from build123d import *

# Parameters (mm, degrees)
SKETCH_1_R          = 39
EXTRUDE_1_DEPTH     = 53.8
SKETCH_2_R          = 2
CUT_EXTRUDE_1_DEPTH = 3
SKETCH_3_R          = 5.25
EXTRUDE_2_DEPTH     = 20
CUT_EXTRUDE_START   = -10
SKETCH_4_R          = 5.5
SKETCH_4_R_2        = 5.25
CUT_EXTRUDE_2_DEPTH = 10
CHAMFER_1_SIZE      = 0.5
CUT_EXTRUDE_3_DEPTH = 10
CHAMFER_2_SIZE      = 1.5
SKETCH_7_W          = 5
SKETCH_7_H          = 9
CUT_EXTRUDE_4_DEPTH = 10
SKETCH_8_W          = 0.130242645
SKETCH_8_H          = 3.5
SKETCH_9_R          = 1.5
CUT_EXTRUDE_5_DEPTH = 10


with BuildPart() as part:
    # 草图1 → 凸台-拉伸1 (new body)
    with BuildSketch(Plane.XY):
        with Locations(Location((0, 0, 0), (0, 0, 180))):
            Circle(SKETCH_1_R)
    extrude(amount=EXTRUDE_1_DEPTH)

    # 草图2 → 切除-拉伸1 (cut)
    with BuildSketch(Plane.XY.offset(53.8)):
        with Locations((0, 20)):
            Circle(SKETCH_2_R)
        with Locations((17.320508076, -10)):
            Circle(SKETCH_2_R)
        with Locations((-17.320508076, -10)):
            Circle(SKETCH_2_R)
    extrude(amount=-CUT_EXTRUDE_1_DEPTH, mode=Mode.SUBTRACT)

    # 草图3 → 凸台-拉伸2 (add)
    with BuildSketch(Plane.XY.offset(53.8)):
        Circle(SKETCH_3_R)
    extrude(amount=EXTRUDE_2_DEPTH)

    # 草图4 → 切除-拉伸2 (cut)
    with BuildSketch(Plane.XY.offset(53.8).offset(CUT_EXTRUDE_START)):
        Circle(SKETCH_4_R)
        Circle(SKETCH_4_R_2, mode=Mode.SUBTRACT)
    extrude(amount=CUT_EXTRUDE_2_DEPTH, mode=Mode.SUBTRACT)

    # 倒角1
    chamfer_1_edges = [part.edges().sort_by_distance(p)[0] for p in [
        (-5.25, 0, 73.8),
    ]]
    chamfer(chamfer_1_edges, length=CHAMFER_1_SIZE)

    # 草图5 → 切除-拉伸3 (cut)
    with BuildSketch(Plane.XY.offset(73.8)):
        Polygon((4.75, 0), (4.75, 11.306536843), (10.594936623, 11.306536843), (10.594936623, -9.408936254), (4.75, -9.408936254), align=None)
    extrude(amount=-CUT_EXTRUDE_3_DEPTH, mode=Mode.SUBTRACT)

    # 倒角2
    chamfer_2_edges = [part.edges().sort_by_distance(p)[0] for p in [
        (39, 0, 53.8),
    ]]
    chamfer(chamfer_2_edges, length=CHAMFER_2_SIZE)

    # 草图6 → 切除-旋转1 (revolve, cut)
    with BuildSketch(Plane(origin=(0, 0, 0), x_dir=(1, 0, 0), z_dir=(0, 1, 0)), mode=Mode.PRIVATE) as cut_revolve_1_sk:
        Polygon((-39, 0), (-39, -1.5), (-33.508685112, 0), align=None)
    revolve(cut_revolve_1_sk.sketch.rotate(Axis((0, 0, 0), (0, 0, -1)), 154.791234703), axis=Axis((0, 0, 0), (0, 0, -1)), mode=Mode.SUBTRACT)

    # 草图7 → 切除-拉伸4 (cut)
    with BuildSketch(Plane(origin=(40, 0, 0), x_dir=(0, 0, -1), z_dir=(1, 0, 0))):
        with Locations((-7, 0)):
            Rectangle(SKETCH_7_W, SKETCH_7_H)
    extrude(amount=-CUT_EXTRUDE_4_DEPTH, mode=Mode.SUBTRACT)

    # 草图8 → 切除-旋转2 (revolve, cut)
    with BuildSketch(Plane(origin=(0, 0, 0), x_dir=(1, 0, 0), z_dir=(0, 1, 0)), mode=Mode.PRIVATE) as cut_revolve_2_sk:
        with Locations((38.934878678, -11.25)):
            Rectangle(SKETCH_8_W, SKETCH_8_H)
    revolve(cut_revolve_2_sk.sketch.rotate(Axis((0, 0, 0), (0, 0, 1)), 25.208765297), axis=Axis((0, 0, 0), (0, 0, 1)), mode=Mode.SUBTRACT)

    # 草图9 → 切除-拉伸5 (cut)
    with BuildSketch(Plane(origin=(4.75, 0, 0), x_dir=(0, 0, -1), z_dir=(1, 0, 0))):
        with Locations((-70.8, 0)):
            Circle(SKETCH_9_R)
    extrude(amount=-CUT_EXTRUDE_5_DEPTH, mode=Mode.SUBTRACT)


solid = part.part
Here's how the part is built. I have some questions about the finished solid (model axes, mm). A direction names the side the tool comes from. Round coordinates to 2 decimals unless told otherwise and drop trailing zeros. Order: outer loops, then holes, each group sorted by start corner. A loop starts at its lowest first (then second) coordinate and runs counter-clockwise, first axis right, second up. Notation, with made-up numbers: (-23, 44) -> (-10, 44) arc R22 ccw to (-10, 59) -> close; hole circle Ø11 at (37.5, 45.25). An arc over 180 degrees is marked (long way). Return JSON: item names as keys, results as strings.
Q1. If we mould it in two halves opening along Z, with no side actions, what happens to faces 4 (the flat face through (34, -4.5, 7)), 5 (the conical face through (10.285, -32.171, 0.073)), 6 (the flat face through (17, -10, 50.8))? For each: released by +Z, released by -Z, zero draft, split by the parting line, or undercut.
Filled sheet:
{"face 4": "undercut", "face 5": "released by -Z", "face 6": "released by +Z"}
Q2. If we section it at C-C on z = 46.5: List the corners of the cut face in (x, y) for me, plus the area to 3 significant figures.
Filled sheet:
{"outline": "circle Ø78 at (0, 0); circle Ø10.5 at (0, 0); hole circle Ø11 at (0, 0)", "area": "4,770 mm^2"}
Q3. For pin 1 Ø1.3 at (y, z) = (0.5, 68.5) entering from +X; pin 2 Ø5 at (y, z) = (-20, 57.5) entering from -X; pin 3 Ø10 at (x, y) = (32.5, 0) entering from +Z; pin 4 Ø4 at (y, z) = (-17, 35) entering from +X, each with a flat end and sliding along its axis, tell me the tip position at first contact or that it passes through.
Filled sheet:
{"pin 1": "stops at x = 4.75", "pin 2": "passes through", "pin 3": "stops at z = 53.8", "pin 4": "stops at x = 36"}
Q4. Which directions (+Z, -Z, +X, -X, +Y, -Y) give clear straight access to the entire face, cutting with the end or side of a thin tool? Please do faces 1 (the cylindrical face through (18.396, -8.314, 52.321)), 2 (the flat face through (4.75, 0, 69)), 3 (the flat face through (30, 0, 7)).
Filled sheet:
{"face 1": "+Z", "face 2": "+Z, +X, +Y, -Y", "face 3": "+X"}
Q5. If we section it at B-B on z = 70.8: List the corners of the cut face in (x, y) for me.
Filled sheet:
{"outline": "(-5.03, -1.5) arc R5.25 ccw to (4.75, -2.24) -> (4.75, -1.5) -> close; (-5.03, 1.5) -> (4.75, 1.5) -> (4.75, 2.24) arc R5.25 ccw to start"}
Q6. I need wall thicknesses on line 1 along Y through (x, z) = (0, 51.7); line 2 along X through (y, z) = (4.5, 48.5); line 3 along Z through (x, y) = (29.5, 13.5). Which ranges of each line are inside material? Lowest first, please. Write a range as from..to.
Filled sheet:
{"line 1": "y = -39..-5.5, -5.25..5.25, 5.5..18, 22..39", "line 2": "x = -38.74..-3.16, -2.7..2.7, 3.16..38.74", "line 3": "z = 0..53.8"}
Q7. If we section it at D-D on z = 17: List the corners of the cut face in (x, y) for me.
Filled sheet:
{"outline": "circle Ø78 at (0, 0)"}
